from build123d import *

# Parameters (mm, degrees)
SKETCH1_R           = 5
BOSS_EXTRUDE1_DEPTH = 2500
SKETCH2_R           = 5
SKETCH2_R_2         = 4.75
CUT_EXTRUDE1_DEPTH  = 49.5
SKETCH3_R           = 4.75
SKETCH3_R_2         = 3
CUT_EXTRUDE2_DEPTH  = 43
CUT_EXTRUDE3_DEPTH  = 6.5
SKETCH6_R           = 3
SKETCH6_R_2         = 2.5
CUT_EXTRUDE4_DEPTH  = 16
CUT_EXTRUDE5_START  = -10
SKETCH7_R           = 5
SKETCH7_R_2         = 3
CUT_EXTRUDE5_DEPTH  = 10


with BuildPart() as part:
    # Sketch1 → Boss-Extrude1 (new body)
    with BuildSketch(Plane.XY):
        Circle(SKETCH1_R)
    extrude(amount=BOSS_EXTRUDE1_DEPTH)

    # Sketch2 → Cut-Extrude1 (cut)
    with BuildSketch(Plane(origin=(0, 0, 0), x_dir=(-1, 0, 0), z_dir=(0, 0, -1))):
        Circle(SKETCH2_R)
        Circle(SKETCH2_R_2, mode=Mode.SUBTRACT)
    extrude(amount=-CUT_EXTRUDE1_DEPTH, mode=Mode.SUBTRACT)

    # Sketch3 → Cut-Extrude2 (cut)
    with BuildSketch(Plane(origin=(0, 0, 0), x_dir=(-1, 0, 0), z_dir=(0, 0, -1))):
        Circle(SKETCH3_R)
        Circle(SKETCH3_R_2, mode=Mode.SUBTRACT)
    extrude(amount=-CUT_EXTRUDE2_DEPTH, mode=Mode.SUBTRACT)

    # Sketch5 → Cut-Extrude3 (cut)
    with BuildSketch(Plane(origin=(0, 0, 43), x_dir=(-1, 0, 0), z_dir=(0, 0, -1))):
        with BuildLine():
            Line((-4, 2.561737691), (-4, -2.561737691))
            ThreePointArc((-4, -2.561737691), (-4.75, 0), (-4, 2.561737691))
        make_face()
        with BuildLine():
            Line((4, 2.561737691), (4, -2.561737691))
            ThreePointArc((4, -2.561737691), (4.75, 0), (4, 2.561737691))
        make_face()
    extrude(amount=-CUT_EXTRUDE3_DEPTH, mode=Mode.SUBTRACT)

    # Sketch6 → Cut-Extrude4 (cut)
    with BuildSketch(Plane(origin=(0, 0, 0), x_dir=(-1, 0, 0), z_dir=(0, 0, -1))):
        Circle(SKETCH6_R)
        Circle(SKETCH6_R_2, mode=Mode.SUBTRACT)
    extrude(amount=-CUT_EXTRUDE4_DEPTH, mode=Mode.SUBTRACT)

    # Sketch7 → Cut-Extrude5 (cut)
    with BuildSketch(Plane.XY.offset(2500).offset(CUT_EXTRUDE5_START)):
        with Locations(Location((0, 0, 0), (0, 0, 180))):
            Circle(SKETCH7_R)
        with Locations(Location((0, 0, 0), (0, 0, 180))):
            Circle(SKETCH7_R_2, mode=Mode.SUBTRACT)
    extrude(amount=CUT_EXTRUDE5_DEPTH, mode=Mode.SUBTRACT)


solid = part.part
Check sheet for the modelled part. Datum: model origin and axes. Units: mm. Give positions to 0.01 mm unless a question says otherwise; leave off trailing zeros. Write each loop counter-clockwise with the first axis right and the second up, starting at its lowest first coordinate (ties: lowest second). Pieces come first, ordered by that corner, then holes. Notation, with made-up numbers: (26, 27) -> (84, 27) arc R11 cw to (84, 35) -> close; hole circle Ø1 at (2.25, 60.5). An arc over 180 degrees is marked (long way). One line per item, written item: value. Start each with the question number.
Item 1: Section check A-A on z = 1308.5. Record the cut outline in (x, y).
Item 2: Material ranges on probe 1 along Y at (x, z) = (3.25, 911); probe 2 along Y at (x, z) = (-0.75, 536); probe 3 along Z at (x, y) = (-3.5, 2.5), recorded low to high. Write a range as from..to.
Item 3: Gauge pin test, flat ends, axial feed: pin 1 (1 mm diameter, centred on y = 1, z = 1441, fed in from -X); pin 2 (2.5 mm diameter, centred on y = 0, z = 47, fed in from -X); pin 3 (2 mm diameter, centred on y = -2.5, z = 2017.5, fed in from +X). Record the tip position at first contact, or that the pin passes through.
Results list:
1. outline: circle Ø10 at (0, 0)
2. probe 1: -3.8..3.8
2. probe 2: -4.94..4.94
2. probe 3: 43..2490
3. pin 1: x = -4.97
3. pin 2: x = -4
3. pin 3: x = 4.77
